Input: dimensioned drawing with shaded views. Units: mm. Origin: part minimum x, y, z. A direction names the side the tool comes from. Give positions to 0.01 mm unless a question says otherwise; leave off trailing zeros. Write each loop counter-clockwise with the first axis right and the second up, starting at its lowest first coordinate (ties: lowest second). Pieces come first, ordered by that corner, then holes. Notation, with made-up numbers: M 69.5,85 L 111.5,85 A14 cw 111.5,101 Z; hole C 59,-37 d9. An arc over 180 degrees is marked long. Answer as a JSON object with one key per item and string values.
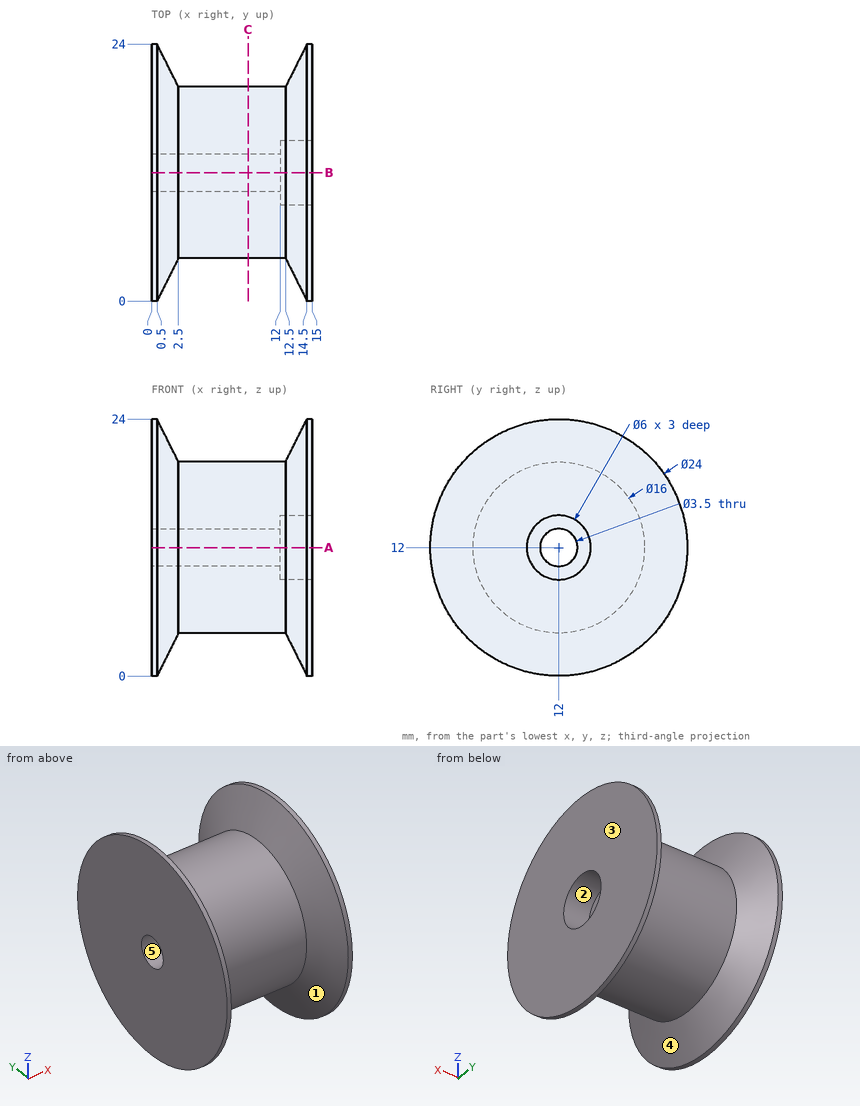
1) Cut plane C-C on x = 9. Return loops of the section in (y, z).
Geometry check:
{"outline": "C 12,12 d16; hole C 12,12 d3.5"}
2) Contact query for flat-ended pins moving along their axis: P1, Ø4, axis at x = 10.5, z = 20, coming from the +Y side; P2, Ø1.5, axis at x = 7.5, z = 15, coming from the +Y side; P3, Ø2, axis at x = 3, y = 13, coming from the -Z side. Output: stop coordinate, or through.
Geometry check:
{"P1": "stops at y = 17.29", "P2": "stops at y = 19.68", "P3": "stops at z = 3.05"}
3) Set-up query: the marked faces 4 and 5. Return all of +Z, -Z, +X, -X, +Y, -Y with unobstructed straight access to the full face (end or side cutting, diameter ignored); none if empty.
Geometry check:
{"face 4": "none", "face 5": "+X, -X"}
4) Cut plane A-A on z = 12. Return loops of the section in (x, y).
Geometry check:
{"outline": "M 0,0 L 0.5,0 L 2.5,4 L 12.5,4 L 14.5,0 L 15,0 L 15,9 L 12,9 L 12,10.25 L 0,10.25 Z; M 0,13.75 L 12,13.75 L 12,15 L 15,15 L 15,24 L 14.5,24 L 12.5,20 L 2.5,20 L 0.5,24 L 0,24 Z"}
5) Pull-direction query (Y, two-part tool) for the marked faces 1, 2 and 3; classes: pulls with the +Y half, pulls with the -Y half, needs draft (parallel to the pull), parting line crosses it, or undercut.
Geometry check:
{"face 1": "parting line crosses it", "face 2": "undercut", "face 3": "needs draft"}
6) Line query: line 1 (Y direction, x = 4.25, z = 12); line 2 (X direction, y = 12.25, z = 21.25); line 3 (Y direction, x = 8.25, z = 13.5). Output: solid intervals per line, ascending. Write a range as from..to.
Geometry check:
{"line 1": "y = 4..10.25, 13.75..20", "line 2": "x = 0..1.87, 13.13..15", "line 3": "y = 4.14..11.1, 12.9..19.86"}
